```python
from build123d import *

# Parameters (mm, degrees)
SKETCH1_W              = 50.8
SKETCH1_H              = 57.15
BOSS_EXTRUDE1_DEPTH    = 12.7
SKETCH2_R              = 11.1125
CUT_EXTRUDE1_DEPTH     = 46.900442536
SKETCH11_W             = 12.7
SKETCH11_H             = 57.15
CUT_EXTRUDE4_DEPTH     = 46.900442536
SKETCH3_W              = 28.575
SKETCH3_H              = 12.7
CUT_EXTRUDE2_DEPTH     = 46.900442536
F_10_CLEARANCE_HOLE1_D = 5.1054
SKETCH6_W              = 3.175
SKETCH6_H              = 37.090012852
CUT_EXTRUDE3_DEPTH     = 24.13
F_10_CLEARANCE_HOLE2_D = 5.1054


with BuildPart() as part:
    # Sketch1 → Boss-Extrude1 (new, symmetric)
    with BuildSketch(Plane(origin=(0, 0, 0), x_dir=(1, 0, 0), z_dir=(0, 1, 0))):
        Rectangle(SKETCH1_W, SKETCH1_H)
    extrude(amount=BOSS_EXTRUDE1_DEPTH, both=True)

    # Sketch2 → Cut-Extrude1 (cut, through all)
    with BuildSketch(Plane(origin=(0, 12.7, 0), x_dir=(1, 0, 0), z_dir=(0, 1, 0))):
        with Locations(Location((-9.525, 0, 0), (0, 0, 270))):
            Circle(SKETCH2_R)
    extrude(amount=-CUT_EXTRUDE1_DEPTH, mode=Mode.SUBTRACT)

    # Sketch11 → Cut-Extrude4 (cut, through all)
    with BuildSketch(Plane(origin=(0, 12.7, 0), x_dir=(1, 0, 0), z_dir=(0, 1, 0))):
        with Locations((19.05, 0)):
            Rectangle(SKETCH11_W, SKETCH11_H)
    extrude(amount=-CUT_EXTRUDE4_DEPTH, mode=Mode.SUBTRACT)

    # Sketch3 → Cut-Extrude2 (cut, through all)
    with BuildSketch(Plane(origin=(0, 12.7, 0), x_dir=(1, 0, 0), z_dir=(0, 1, 0))):
        with Locations((-1.5875, 22.225)):
            Rectangle(SKETCH3_W, SKETCH3_H)
        with Locations((-1.5875, -22.225)):
            Rectangle(SKETCH3_W, SKETCH3_H)
    extrude(amount=-CUT_EXTRUDE2_DEPTH, mode=Mode.SUBTRACT)

    # #10 Clearance Hole1 (through all)
    with Locations(Plane(origin=(-15.875, 0, 0), x_dir=(0, 0, -1), z_dir=(1, 0, 0))):
        with Locations((22.225, 0), (-22.225, 0)):
            Hole(F_10_CLEARANCE_HOLE1_D / 2)

    # Sketch6 → Cut-Extrude3 (cut)
    with BuildSketch(Plane(origin=(12.7, 0, 0), x_dir=(0, 0, -1), z_dir=(1, 0, 0))):
        Rectangle(SKETCH6_W, SKETCH6_H)
    extrude(amount=-CUT_EXTRUDE3_DEPTH, mode=Mode.SUBTRACT)

    # #10 Clearance Hole2 (through all)
    with Locations(Plane.XY.offset(15.875)):
        with Locations((6.985, 0)):
            Hole(F_10_CLEARANCE_HOLE2_D / 2)


solid = part.part
```
Geometry check sheet. Reference: the model listing, model coordinates, mm. A direction names the side the tool comes from. Round coordinates to 2 decimals unless told otherwise and drop trailing zeros. Order: outer loops, then holes, each group sorted by start corner. A loop starts at its lowest first (then second) coordinate and runs counter-clockwise, first axis right, second up. Notation, with made-up numbers: (-19.5, 36) -> (-6.5, 36) arc R28 cw to (-6.5, 64) -> close; hole circle Ø10 at (55.25, 37.25). An arc over 180 degrees is marked (long way). Return JSON: item names as keys, results as strings. Group by question number.
Q1. Section check D-D, the plane y = 7.5. Record the boundary of the cut face in (x, z) (1 decimal).
Q2. Section check C-C, the plane x = -11.5. Record the boundary of the cut face in (y, z) (3 decimals), plus the area to 3 significant figures.
Q3. Release check for a two-part mould opening along Y. For faces 1 (the flat face through (-2, 0, -15.875)), 2 (the flat face through (-19, 12.7, -7)), 3 (the cylindrical face through (-20.704, 0.112, -24.775)) record: released by +Y, released by -Y, zero draft, split by the parting line, or undercut.
Q4. Gauge pin test, flat ends, axial feed: pin 1 (1 mm diameter, centred on x = -11, y = -10, fed in from +Z) (3 decimals); pin 2 (8 mm diameter, centred on y = 0, z = -22.225, fed in from +X) (3 decimals); pin 3 (7.5 mm diameter, centred on x = -5.5, y = -1.5, fed in from -Z) (3 decimals). Record the tip position at first contact, or that the pin passes through.
Q5. Section check B-B, the plane z = -3. Record the boundary of the cut face in (x, y) (3 decimals), plus the area to 3 significant figures.
Q6. Tool access check on faces 4 (the flat face through (-15.875, 0, -19)), 5 (the flat face through (-2, 0, 15.875)), 6 (the flat face through (10, 0, 1.588)). Record the directions out of +Z, -Z, +X, -X, +Y, -Y that give a thin tool (end or side, any length) a straight path to the whole face; none if there is none.
Q7. Section check A-A, the plane y = 0. Record the boundary of the cut face in (x, z) (1 decimal).
Q8. Material ranges on probe 1 along Z at (x, y) = (9.5, -5.75) (1 decimal); probe 2 along X at (y, z) = (2.5, 25) (3 decimals); probe 3 along Z at (x, y) = (-3.5, -10.75) (3 decimals), recorded low to high. Write a range as from..to.
Numbers:
{
 "1": {"outline": "(-25.4, -28.6) -> (-15.9, -28.6) -> (-15.9, -15.9) -> (12.7, -15.9) -> (12.7, -1.6) -> (1.5, -1.6) arc R11.1 cw (long way) to (1.5, 1.6) -> (12.7, 1.6) -> (12.7, 15.9) -> (-15.9, 15.9) -> (-15.9, 28.6) -> (-25.4, 28.6) -> close"},
 "2": {"outline": "(-12.7, -15.875) -> (12.7, -15.875) -> (12.7, -10.936) -> (-12.7, -10.936) -> close; (-12.7, 10.936) -> (12.7, 10.936) -> (12.7, 15.875) -> (-12.7, 15.875) -> close", "area": "251 mm^2"},
 "3": {"face 1": "zero draft", "face 2": "released by +Y", "face 3": "undercut"},
 "4": {"pin 1": "z = 15.875", "pin 2": "x = -15.875", "pin 3": "z = -15.875"},
 "5": {"outline": "(-25.4, -12.7) -> (-20.225, -12.7) -> (-20.225, 12.7) -> (-25.4, 12.7) -> close; (1.175, -12.7) -> (12.7, -12.7) -> (12.7, 12.7) -> (1.175, 12.7) -> close; hole circle Ø5.105 at (6.985, 0)", "area": "404 mm^2"},
 "6": {"face 4": "-Z, +X, +Y, -Y", "face 5": "+Z, +X, +Y, -Y", "face 6": "+X, +Y, -Y"},
 "7": {"outline": "(-25.4, -28.6) -> (-15.9, -28.6) -> (-15.9, -24.8) -> (-25.4, -24.8) -> close; (-25.4, -19.7) -> (-15.9, -19.7) -> (-15.9, -15.9) -> (4.4, -15.9) -> (4.4, -1.6) -> (1.5, -1.6) arc R11.1 cw (long way) to (1.5, 1.6) -> (4.4, 1.6) -> (4.4, 15.9) -> (-15.9, 15.9) -> (-15.9, 19.7) -> (-25.4, 19.7) -> close; (-25.4, 24.8) -> (-15.9, 24.8) -> (-15.9, 28.6) -> (-25.4, 28.6) -> close; (9.5, -15.9) -> (12.7, -15.9) -> (12.7, -1.6) -> (9.5, -1.6) -> close; (9.5, 1.6) -> (12.7, 1.6) -> (12.7, 15.9) -> (9.5, 15.9) -> close"},
 "8": {"probe 1": "-15.9..-1.6, 1.6..15.9", "probe 2": "-25.4..-15.875", "probe 3": "-15.875..-9.337, 9.337..15.875"}
}
